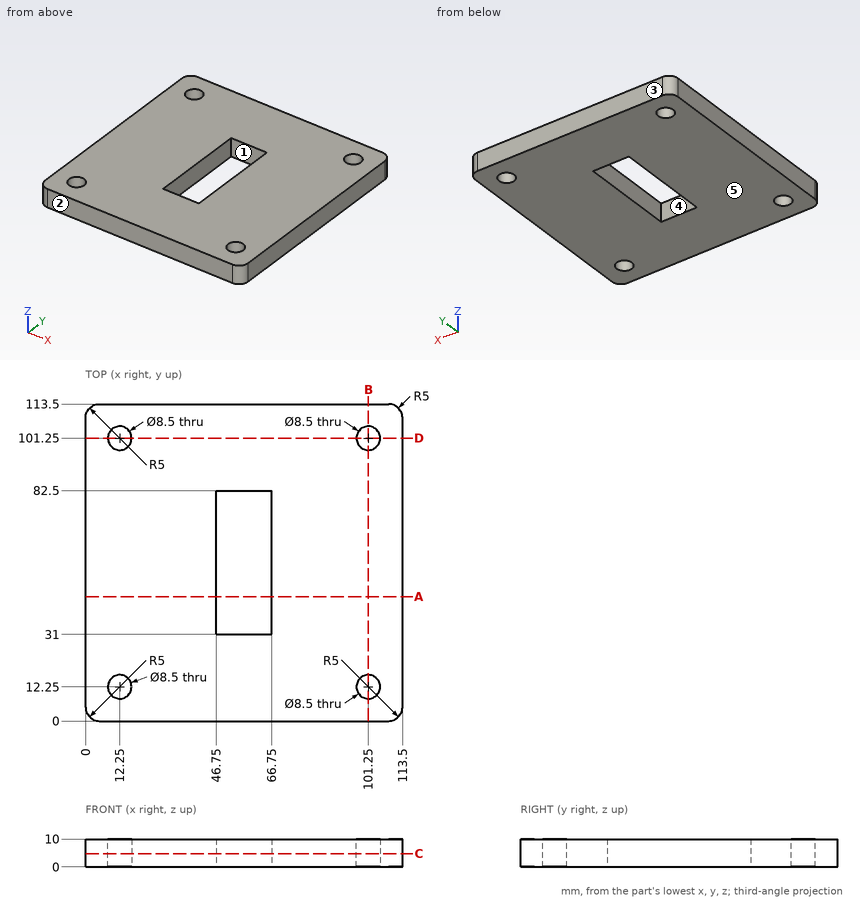
Study the drawing (mm; zero at the part's minimum x, y, z) and answer. A direction names the side the tool comes from. Round coordinates to 2 decimals unless told otherwise and drop trailing zeros. Order: outer loops, then holes, each group sorted by start corner. A loop starts at its lowest first (then second) coordinate and runs counter-clockwise, first axis right, second up. Notation, with made-up numbers: (-22.75, -38.75) - (12.25, -38.75) arc R19 cw to (12.25, -28.75) - close; hole circle Ø1 at (-10, -37.75). An arc over 180 degrees is marked (long way). Use one line per item in the form item = value. Start each with the question number.
(1) A flat-ended cylindrical pin translates along its axis: pin 1 Ø13.5 at (x, y) = (101.25, 12.25) entering from +Z. Find the tip coordinate at first contact, or state that the pin passes through.
(2) The part is cut by section B-B (x = 101.25). Give the vertices of the cut face in (y, z), then the cut area to 3 significant figures.
(3) Find the intervals of material crossed by line 1 along Y through (x, z) = (12.25, 2.75); line 2 along Y through (x, z) = (47, 0.75); line 3 along X through (y, z) = (49, 6.25), in increasing order. Write a range as from..to.
(4) For the marked faces 4 and 5, determine the directions among +Z, -Z, +X, -X, +Y, -Y from which every point of the face is accessible in a straight line to the end or side of a thin tool.
(5) The part is cut by section A-A (y = 44.5). Give the vertices of the cut face in (x, z), then the cut area to 3 significant figures.
(6) The part is cut by section C-C (z = 4.75). Give the vertices of the cut face in (x, y), then the cut area to 3 significant figures.
(7) Determine the mould class of the marked faces 1, 2 and 3 for opening direction Y: +Y half, -Y half, draft (parallel to the pull), parting line (faces both ways), or undercut.
Checked values:
q1.pin_1 = 10
q2.outline = (0, 0) - (8, 0) - (8, 10) - (0, 10) - close; (16.5, 0) - (97, 0) - (97, 10) - (16.5, 10) - close; (105.5, 0) - (113.5, 0) - (113.5, 10) - (105.5, 10) - close
q2.area = 965 mm^2
q3.line_1 = 0..8, 16.5..97, 105.5..113.5
q3.line_2 = 0..31, 82.5..113.5
q3.line_3 = 0..46.75, 66.75..113.5
q4.face_4 = +Z, -Z
q4.face_5 = -Z, +X, -X, +Y, -Y
q5.outline = (0, 0) - (46.75, 0) - (46.75, 10) - (0, 10) - close; (66.75, 0) - (113.5, 0) - (113.5, 10) - (66.75, 10) - close
q5.area = 935 mm^2
q6.outline = (0, 5) arc R5 ccw to (5, 0) - (108.5, 0) arc R5 ccw to (113.5, 5) - (113.5, 108.5) arc R5 ccw to (108.5, 113.5) - (5, 113.5) arc R5 ccw to (0, 108.5) - close; hole circle Ø8.5 at (12.25, 12.25); hole circle Ø8.5 at (12.25, 101.25); hole (46.75, 31) - (66.75, 31) - (66.75, 82.5) - (46.75, 82.5) - close; hole circle Ø8.5 at (101.25, 12.25); hole circle Ø8.5 at (101.25, 101.25)
q6.area = 11,600 mm^2
q7.face_1 = undercut
q7.face_2 = -Y half
q7.face_3 = +Y half
